Build history of the part. All positions in model axes, mm. Give positions to 0.01 mm unless a question says otherwise; leave off trailing zeros. Order: outer loops, then holes, each group sorted by start corner. A loop starts at its lowest first (then second) coordinate and runs counter-clockwise, first axis right, second up. Notation, with made-up numbers: M 22,75 L 40,75 A13 ccw 40,79 Z; hole C 77.25,66.25 d4. An arc over 180 degrees is marked long. One line per item, written item: value.
from build123d import *

# Parameters (mm, degrees)
SKETCH1_W           = 10
SKETCH1_H           = 35
SKETCH1_R           = 1.5
BOSS_EXTRUDE1_DEPTH = 10
FILLET1_R           = 5
FILLET2_R           = 5


with BuildPart() as part:
    # Sketch1 → Boss-Extrude1 (new body)
    with BuildSketch(Plane.XY):
        with Locations((5, 17.5)):
            Rectangle(SKETCH1_W, SKETCH1_H)
        with Locations((5, 25)):
            Circle(SKETCH1_R, mode=Mode.SUBTRACT)
        with Locations((5, 5)):
            Circle(SKETCH1_R, mode=Mode.SUBTRACT)
    extrude(amount=BOSS_EXTRUDE1_DEPTH)

    # Fillet1
    # the kernel refuses this fillet: 5 mm, written as the material it takes off along each edge
    with BuildSketch(Plane(origin=(-12.5, 0, 10), x_dir=(0, 0, -1), z_dir=(1, 0, 0))) as fillet1_piece_1:
        with BuildLine():
            CenterArc((FILLET1_R, FILLET1_R), FILLET1_R, 180, 90)
            Line((0, FILLET1_R), (0, 0))
            Line((0, 0), (FILLET1_R, 0))
        make_face()
    extrude(amount=35, mode=Mode.SUBTRACT)

    # Fillet2
    fillet2_edges = [part.edges().sort_by_distance(p)[0] for p in [
        (5, 35, 10),
    ]]
    fillet(fillet2_edges, radius=FILLET2_R)


solid = part.part
1) Drill centre lines: probe 1 along Y at (x, z) = (5, 3.75); probe 2 along Y at (x, z) = (5, 6.25); probe 3 along X at (y, z) = (24, 5.5). Where is each one in solid material? Low to high. Write a range as from..to.
Check values:
probe 1: 0..3.5, 6.5..23.5, 26.5..35
probe 2: 0.16..3.5, 6.5..23.5, 26.5..34.84
probe 3: 0..3.88, 6.12..10
2) Saw through at A-A, the plane y = 25. Write the cut outline in (x, z).
Check values:
outline: M 0,0 L 3.5,0 L 3.5,10 L 0,10 Z; M 6.5,0 L 10,0 L 10,10 L 6.5,10 Z
3) Pin check, flat tips, straight feed: pin 1 (1.5 mm diameter, centred on x = 6, z = 3.5, fed in from -Y); pin 2 (2.5 mm diameter, centred on x = 5, y = 5, fed in from -Z). Stop position of each tip, or through.
Check values:
pin 1: y = 0
pin 2: through
4) Saw through at B-B, the plane z = 9. Write the cut outline in (x, y).
Check values:
outline: M 0,2 L 10,2 L 10,33 L 0,33 Z; hole C 5,5 d3; hole C 5,25 d3
5) Saw through at C-C, the plane x = 5. Write the cut outline in (y, z).
Check values:
outline: M 0,0 L 3.5,0 L 3.5,9.77 A5 ccw 0,5 Z; M 6.5,0 L 23.5,0 L 23.5,10 L 6.5,10 Z; M 26.5,0 L 35,0 L 35,5 A5 ccw 30,10 L 26.5,10 Z
6) Saw through at D-D, the plane x = 3. Write the cut outline in (y, z), then the cut area to 3 significant figures.
Check values:
outline: M 0,0 L 35,0 L 35,5 A5 ccw 30,10 L 5,10 A5 ccw 0,5 Z
area: 339 mm^2
7) Mould opens along X. For faces 1 (the face through (5, 18, 10)), 2 (the face through (4.805, 26.487, 4.93)), 3 (the face through (10, 17, 5)) say: released by +X, released by -X, zero draft, split by the parting line, or undercut.
Check values:
face 1: zero draft
face 2: undercut
face 3: released by +X
